Part model, mm, in its own coordinate system. A direction names the side the tool comes from. Round coordinates to 2 decimals unless told otherwise and drop trailing zeros. Loops run counter-clockwise (first coordinate to the right, second up) from the corner with the lowest first, then second, coordinate; pieces in that order, holes last. Notation, with made-up numbers: (41, -9) -> (45, -9) arc R20 cw to (45, 3) -> close; hole circle Ø1 at (71.5, 36.25). An arc over 180 degrees is marked (long way). Use a Markdown table: item, result. Add a question column.
Item 1: Which spindle directions (+Z, -Z, +X, -X, +Y, -Y) get a long thin tool onto all of the face, cutting with end or side? Do faces 1 (the face through (19, 2, -30)), 2 (the face through (34.4, 1.52, -34.43)). Say none if no direction does.
Item 2: Two-plate mould, pull along Z, no slides. Class faces 3 (the face through (-35, 1, 0)), 4 (the face through (31, 1, 35)), 5 (the face through (31.3, 1.5, 33.4)), 6 (the face through (-33.7, 1.5, -31.6)): pulls with the +Z half, pulls with the -Z half, needs draft (parallel to the pull), parting line crosses it, or undercut.
Item 3: Cut at B-B, the plane y = 1.3. List the corners of the cut face in (x, z), plus the area to 3 significant figures.
Item 4: Cut at A-A, the plane z = 27.5. List the corners of the cut face in (x, y), plus the area to 3 significant figures.
Item 5: Flat gauge pin, fed straight in: pin 1 (3.5 mm diameter, centred on x = -32.5, z = -32.5, fed in from +Y). Where does the tip first touch, or does it go through?
Item 6: Probe line 1 (X direction, y = 1.3, z = 32.5); line 2 (Z direction, x = -32.5, y = 2.3); line 3 (X direction, y = 1.05, z = -9). List the from-to ranges inside material, lowest first. Write a range as [from, to].
Item 7: Cut at C-C, the plane x = 25.5. List the corners of the cut face in (y, z), plus the area to 3 significant figures.
```python
from build123d import *

# Parameters (mm, degrees)
SKETCH1_W           = 70
SKETCH1_H           = 70
SKETCH1_R           = 1.5
BOSS_EXTRUDE1_DEPTH = 3
FILLET1_R           = 2
SKETCH2_W           = 21.6
SKETCH2_H           = 70
CUT_EXTRUDE2_DEPTH  = 10


with BuildPart() as part:
    # Sketch1 → Boss-Extrude1 (new body)
    with BuildSketch(Plane(origin=(0, 0, 0), x_dir=(1, 0, 0), z_dir=(0, 1, 0))):
        Rectangle(SKETCH1_W, SKETCH1_H)
        with Locations((-32.5, 32.5)):
            Circle(SKETCH1_R, mode=Mode.SUBTRACT)
        with Locations((32.5, 32.5)):
            Circle(SKETCH1_R, mode=Mode.SUBTRACT)
        with Locations((32.5, -32.5)):
            Circle(SKETCH1_R, mode=Mode.SUBTRACT)
        with Locations((-32.5, -32.5)):
            Circle(SKETCH1_R, mode=Mode.SUBTRACT)
    extrude(amount=BOSS_EXTRUDE1_DEPTH)

    # Fillet1
    fillet1_edges = [part.edges().sort_by_distance(p)[0] for p in [
        (35, 1.5, 35),
        (-35, 1.5, 35),
        (-35, 1.5, -35),
        (35, 1.5, -35),
    ]]
    fillet(fillet1_edges, radius=FILLET1_R)

    # Sketch2 → Cut-Extrude2 (cut)
    with BuildSketch(Plane(origin=(0, 3, 0), x_dir=(1, 0, 0), z_dir=(0, 1, 0))):
        with Locations((19.2, -5)):
            Rectangle(SKETCH2_W, SKETCH2_H)
    extrude(amount=-CUT_EXTRUDE2_DEPTH, mode=Mode.SUBTRACT)


solid = part.part
```
A:
| question | item | result |
|---|---|---|
| 1 | face 1 | +Z, +Y, -Y |
| 1 | face 2 | -Z, +X, +Y, -Y |
| 2 | face 3 | needs draft |
| 2 | face 4 | pulls with the +Z half |
| 2 | face 5 | undercut |
| 2 | face 6 | undercut |
| 3 | outline | (-35, -33) arc R2 ccw to (-33, -35) -> (33, -35) arc R2 ccw to (35, -33) -> (35, 33) arc R2 ccw to (33, 35) -> (30, 35) -> (30, -30) -> (8.4, -30) -> (8.4, 35) -> (-33, 35) arc R2 ccw to (-35, 33) -> close; hole circle Ø3 at (-32.5, -32.5); hole circle Ø3 at (-32.5, 32.5); hole circle Ø3 at (32.5, -32.5); hole circle Ø3 at (32.5, 32.5) |
| 3 | area | 3,460 mm^2 |
| 4 | outline | (-35, 0) -> (8.4, 0) -> (8.4, 3) -> (-35, 3) -> close; (30, 0) -> (35, 0) -> (35, 3) -> (30, 3) -> close |
| 4 | area | 145 mm^2 |
| 5 | pin 1 | stops at y = 3 |
| 6 | line 1 | x = [-35, -34], [-31, 8.4], [30, 31], [34, 35] |
| 6 | line 2 | z = [-35, -34], [-31, 31], [34, 35] |
| 6 | line 3 | x = [-35, 8.4], [30, 35] |
| 7 | outline | (0, -35) -> (3, -35) -> (3, -30) -> (0, -30) -> close |
| 7 | area | 15.0 mm^2 |
